from build123d import *

# Parameters (mm, degrees)
F1_DEPTH = 25
F3_DEPTH = 23
F4_R     = 1.25
F5_DEPTH = 3
F6_R     = 1.25
F7_DEPTH = 3


with BuildPart() as f1:
    # F0 (on Top) → F1 (new body)
    with BuildSketch(Plane.XY):
        with BuildLine():
            ThreePointArc((-70.7106781187, 70.7106781187), (-38.2683432365, 92.3879532511), (0, 100))
            Line((0, 100), (0, 124.899959968))
            ThreePointArc((0, 124.899959968), (-1.5358983849, 128.5055112434), (-5.2, 129.8959583667))
            ThreePointArc((-5.2, 129.8959583667), (-49.7488462075, 120.1043392265), (-88.1733577476, 95.527268272))
            ThreePointArc((-88.1733577476, 95.527268272), (-89.7810742569, 91.9531625832), (-88.3176086633, 88.3176086633))
            Line((-88.3176086633, 88.3176086633), (-70.7106781187, 70.7106781187))
        make_face()
    extrude(amount=F1_DEPTH)

    # F2 (on face) → F3 (cut)
    with BuildSketch(Plane(origin=(0, 0, 0), x_dir=(1, 0, 0), z_dir=(0, 0, -1))):
        with BuildLine():
            ThreePointArc((-86.1962913084, -90.4389260182), (-86.7816787829, -91.8931506594), (-86.1385908202, -93.3227959561))
            ThreePointArc((-86.1385908202, -93.3227959561), (-48.6007975278, -117.3327045338), (-5.0800001691, -126.8983635506))
            ThreePointArc((-5.0800001691, -126.8983635506), (-3.6143564257, -126.342183526), (-2.9999957734, -124.899959968))
            Line((-2.9999957734, -124.899959968), (-2.9999957734, -102.9562973047))
            Line((-2.9999957734, -102.9562973047), (-2.9999957734, -99.9549899973))
            ThreePointArc((-2.9999957734, -99.9549899973), (-38.2683432365, -92.3879532511), (-68.5575338856, -72.8001685954))
            Line((-68.5575338856, -72.8001685954), (-70.6797786351, -74.9224133449))
            Line((-70.6797786351, -74.9224133449), (-86.1962913084, -90.4389260182))
        make_face()
    extrude(amount=-F3_DEPTH, mode=Mode.SUBTRACT)

    # F4 (on face) → F5 (cut)
    with BuildSketch(Plane(origin=(0, 0, 0), x_dir=(0.7071067812, -0.7071067812, 0), z_dir=(-0.7071067812, -0.7071067812, 0))):
        with Locations((-105, 20)):
            Circle(F4_R)
        with Locations((-105, 15)):
            Circle(F4_R)
        with Locations((-105, 10)):
            Circle(F4_R)
        with Locations((-105, 5)):
            Circle(F4_R)
        with Locations((-110, 20)):
            Circle(F4_R)
        with Locations((-110, 15)):
            Circle(F4_R)
        with Locations((-110, 10)):
            Circle(F4_R)
        with Locations((-110, 5)):
            Circle(F4_R)
        with Locations((-115, 20)):
            Circle(F4_R)
        with Locations((-115, 15)):
            Circle(F4_R)
        with Locations((-115, 10)):
            Circle(F4_R)
        with Locations((-115, 5)):
            Circle(F4_R)
        with Locations((-120, 20)):
            Circle(F4_R)
        with Locations((-120, 15)):
            Circle(F4_R)
        with Locations((-120, 10)):
            Circle(F4_R)
        with Locations((-120, 5)):
            Circle(F4_R)
    extrude(amount=-F5_DEPTH, mode=Mode.SUBTRACT)

    # F6 (on face) → F7 (cut)
    with BuildSketch(Plane.YZ):
        with Locations((105, 20)):
            Circle(F6_R)
        with Locations((105, 15)):
            Circle(F6_R)
        with Locations((105, 10)):
            Circle(F6_R)
        with Locations((105, 5)):
            Circle(F6_R)
        with Locations((110, 20)):
            Circle(F6_R)
        with Locations((110, 15)):
            Circle(F6_R)
        with Locations((110, 10)):
            Circle(F6_R)
        with Locations((110, 5)):
            Circle(F6_R)
        with Locations((115, 20)):
            Circle(F6_R)
        with Locations((115, 15)):
            Circle(F6_R)
        with Locations((115, 10)):
            Circle(F6_R)
        with Locations((115, 5)):
            Circle(F6_R)
        with Locations((120, 20)):
            Circle(F6_R)
        with Locations((120, 15)):
            Circle(F6_R)
        with Locations((120, 10)):
            Circle(F6_R)
        with Locations((120, 5)):
            Circle(F6_R)
    extrude(amount=-F7_DEPTH, mode=Mode.SUBTRACT)


solid = f1.part
Part model, mm, in its own coordinate system. A direction names the side the tool comes from. Round coordinates to 2 decimals unless told otherwise and drop trailing zeros. Order: outer loops, then holes, each group sorted by start corner. A loop starts at its lowest first (then second) coordinate and runs counter-clockwise, first axis right, second up. Notation, with made-up numbers: (19, 78.5) -> (35, 78.5) arc R23 ccw to (35, 88.5) -> close; hole circle Ø7 at (2, 78). An arc over 180 degrees is marked (long way). Put each result on its own line as item: value.
Q1. Band-saw the part on D-D (y = 105). Give the cut face in (x, z), and give its area (3 significant figures).
From the geometry:
outline: (-76.65, 0) -> (-71.44, 0) -> (-71.44, 23) -> (-3, 23) -> (-3, 21.25) -> (0, 21.25) -> (0, 25) -> (-76.65, 25) -> close; (-3, 0) -> (0, 0) -> (0, 3.75) -> (-3, 3.75) -> close; (-3, 6.25) -> (0, 6.25) -> (0, 8.75) -> (-3, 8.75) -> close; (-3, 11.25) -> (0, 11.25) -> (0, 13.75) -> (-3, 13.75) -> close; (-3, 16.25) -> (0, 16.25) -> (0, 18.75) -> (-3, 18.75) -> close
area: 312 mm2
Q2. Wall check: line 1 (Z direction, x = -1.55, y = 115); line 2 (Z direction, x = -16.5, y = 123); line 3 (X direction, y = 108, z = 7.25). Give the ranges that are in metal, low to high. Write a range as [from, to].
From the geometry:
line 1: z = [0, 3.75], [6.25, 8.75], [11.25, 13.75], [16.25, 18.75], [21.25, 25]
line 2: z = [23, 25]
line 3: x = [-72.36, -66.82], [-3, 0]
Q3. Band-saw the part on B-B (y = 115). Give the cut face in (x, z).
From the geometry:
outline: (-60.62, 0) -> (-53.89, 0) -> (-53.89, 23) -> (-3, 23) -> (-3, 21.25) -> (0, 21.25) -> (0, 25) -> (-60.62, 25) -> close; (-3, 0) -> (0, 0) -> (0, 3.75) -> (-3, 3.75) -> close; (-3, 6.25) -> (0, 6.25) -> (0, 8.75) -> (-3, 8.75) -> close; (-3, 11.25) -> (0, 11.25) -> (0, 13.75) -> (-3, 13.75) -> close; (-3, 16.25) -> (0, 16.25) -> (0, 18.75) -> (-3, 18.75) -> close
Q4. Tool access for faces 4 (the face through (-1.479, 121.155, 19.521)), 5 (the face through (-76.261, 78.352, 16.054)), 6 (the face through (-77.253, 81.496, 11.339)): list every direction of +Z, -Z, +X, -X, +Y, -Y with a clear straight run to the whole face (end or side of a thin tool).
From the geometry:
face 4: +X
face 5: none
face 6: -Z, +X
Q5. Pin check, flat tips, straight feed: pin 1 Ø1.5 at (y, z) = (89.5, 3.5) entering from -X; pin 2 Ø2 at (y, z) = (110, 20) entering from -X; pin 3 Ø1.5 at (y, z) = (115, 5) entering from -X. Stop position of each tip, or through.
From the geometry:
pin 1: stops at x = -89.52
pin 2: stops at x = -70.84
pin 3: stops at x = -62.02
Q6. Band-saw the part on A-A (z = 17.5). Give the cut face in (x, y).
From the geometry:
outline: (-88.32, 88.32) -> (-70.71, 70.71) arc R100 cw to (-68.56, 72.8) -> (-86.2, 90.44) arc R2 cw to (-86.14, 93.32) arc R127 cw to (-5.08, 126.9) arc R2 cw to (-3, 124.9) -> (-3, 99.95) arc R100 cw to (0, 100) -> (0, 124.9) arc R5 ccw to (-5.2, 129.9) arc R130 ccw to (-88.17, 95.53) arc R5 ccw to start
Q7. Pull direction Y, two halves, no side cores. Call faces 1 (the face through (-1.5, 128.47, 12.32)), 2 (the face through (-1.48, 106.19, 15.38)), 3 (the face through (-89.78, 92.01, 12.32)): pulls with the +Y half, pulls with the -Y half, needs draft (parallel to the pull), parting line crosses it, or undercut.
From the geometry:
face 1: pulls with the +Y half
face 2: undercut
face 3: parting line crosses it
Q8. Band-saw the part on C-C (x = -66.5). Give the cut face in (y, z).
From the geometry:
outline: (74.68, 23) -> (108.2, 23) -> (108.2, 0) -> (111.7, 0) -> (111.7, 25) -> (74.68, 25) -> close
